```python
from build123d import *

# Parameters (mm, degrees)
SKETCH1_W            = 127
SKETCH1_H            = 25.4
BOSS_EXTRUDE1_DEPTH  = 4.7625
SKETCH2_W            = 4.7625
SKETCH2_H            = 25.4
SKETCH2_H_2          = 12.7
BOSS_EXTRUDE2_DEPTH  = 44.45
SKETCH3_W            = 25.4
SKETCH3_H            = 4.7625
BOSS_EXTRUDE3_DEPTH  = 7.9375
SKETCH4_W            = 12.7
SKETCH4_H            = 4.7625
BOSS_EXTRUDE4_DEPTH  = 7.9375
FILLET1_R            = 6.35
FILLET1_OF_MIRROR1_R = 6.35
SKETCH5_W            = 127
SKETCH5_H            = 2.0955
CUT_EXTRUDE1_DEPTH   = 5.08
SKETCH6_W            = 127
SKETCH6_H            = 1.5875
BOSS_EXTRUDE5_DEPTH  = 5.08


with BuildPart() as part:
    # Sketch1 → Boss-Extrude1 (new body)
    with BuildSketch(Plane(origin=(0, 0, 0), x_dir=(1, 0, 0), z_dir=(0, 1, 0))):
        with Locations((63.5, 12.7)):
            Rectangle(SKETCH1_W, SKETCH1_H)
    extrude(amount=BOSS_EXTRUDE1_DEPTH)

    # Sketch2 → Boss-Extrude2 (add)
    with BuildSketch(Plane(origin=(0, 4.7625, 0), x_dir=(1, 0, 0), z_dir=(0, 1, 0))):
        with Locations((42.06875, 12.7)):
            Rectangle(SKETCH2_W, SKETCH2_H)
        with Locations((16.66875, 6.35)):
            Rectangle(SKETCH2_W, SKETCH2_H_2)
    boss_extrude2 = extrude(amount=BOSS_EXTRUDE2_DEPTH)

    # Sketch3 → Boss-Extrude3 (add)
    with BuildSketch(Plane(origin=(44.45, 0, 0), x_dir=(0, 0, -1), z_dir=(1, 0, 0))):
        with Locations((12.7, 46.83125)):
            Rectangle(SKETCH3_W, SKETCH3_H)
    boss_extrude3 = extrude(amount=BOSS_EXTRUDE3_DEPTH)

    # Sketch4 → Boss-Extrude4 (add)
    with BuildSketch(Plane(origin=(19.05, 0, 0), x_dir=(0, 0, -1), z_dir=(1, 0, 0))):
        with Locations((6.35, 46.83125)):
            Rectangle(SKETCH4_W, SKETCH4_H)
    boss_extrude4 = extrude(amount=BOSS_EXTRUDE4_DEPTH)

    # Fillet1
    fillet1_edges = [part.edges().sort_by_distance(p)[0] for p in [
        (39.6875, 4.7625, -12.7),
        (44.45, 4.7625, -12.7),
        (19.05, 4.7625, -6.35),
        (14.2875, 4.7625, -6.35),
        (44.45, 44.45, -12.7),
        (19.05, 44.45, -6.35),
    ]]
    fillet(fillet1_edges, radius=FILLET1_R)

    # Mirror1: Boss-Extrude2, Boss-Extrude3, Boss-Extrude4 across plane
    add(boss_extrude2.mirror(Plane(origin=(63.5, 0, 0), x_dir=(0, 0, 1), z_dir=(1, 0, 0))))
    add(boss_extrude3.mirror(Plane(origin=(63.5, 0, 0), x_dir=(0, 0, 1), z_dir=(1, 0, 0))))
    add(boss_extrude4.mirror(Plane(origin=(63.5, 0, 0), x_dir=(0, 0, 1), z_dir=(1, 0, 0))))

    # Fillet1 of Mirror1
    fillet1_of_mirror1_edges = [part.edges().sort_by_distance(p)[0] for p in [
        (87.3125, 4.7625, -12.7),
        (82.55, 4.7625, -12.7),
        (107.95, 4.7625, -6.35),
        (112.7125, 4.7625, -6.35),
        (82.55, 44.45, -12.7),
        (107.95, 44.45, -6.35),
    ]]
    fillet(fillet1_of_mirror1_edges, radius=FILLET1_OF_MIRROR1_R)

    # Sketch5 → Cut-Extrude1 (cut)
    with BuildSketch(Plane.XY):
        with Locations((63.5, 2.38125)):
            Rectangle(SKETCH5_W, SKETCH5_H)
    extrude(amount=-CUT_EXTRUDE1_DEPTH, mode=Mode.SUBTRACT)

    # Sketch6 → Boss-Extrude5 (add)
    with BuildSketch(Plane(origin=(0, 0, -25.4), x_dir=(-1, 0, 0), z_dir=(0, 0, -1))):
        with Locations((-63.5, 2.38125)):
            Rectangle(SKETCH6_W, SKETCH6_H)
    extrude(amount=BOSS_EXTRUDE5_DEPTH)


solid = part.part
```
CAD build for the part. Positions are in the model's coordinates, mm. A direction names the side the tool comes from. Round coordinates to 2 decimals unless told otherwise and drop trailing zeros. Write each loop counter-clockwise with the first axis right and the second up, starting at its lowest first coordinate (ties: lowest second). Pieces come first, ordered by that corner, then holes. Notation, with made-up numbers: (-8.5, 60) - (32.5, 60) arc R25 cw to (32.5, 81) - close; hole circle Ø3 at (9, 9.5). An arc over 180 degrees is marked (long way). Return JSON: item names as keys, results as strings. Group by question number.
Item 1: Probe probe 1 along X at (y, z) = (26, -12); probe 2 along Y at (x, z) = (29.5, -2); probe 3 along X at (y, z) = (22, -14). List the from-to ranges inside material, lowest first.
Item 2: Band-saw the part on C-C on x = 90. List the corners of the cut face in (y, z) (1 decimal), plus the area to 3 significant figures.
Item 3: Band-saw the part on B-B on z = -17. List the corners of the cut face in (x, y).
Item 4: Band-saw the part on A-A on x = 54.5. List the corners of the cut face in (y, z) (1 decimal).
Item 5: 3-axis set-ups, long thin cutter, end or side, ignore diameter. For faces 1 (the face through (107.95, 24, -6)), 2 (the face through (64, 4, -25.4)), 3 (the face through (112.712, 30, -6)): which of +Z, -Z, +X, -X, +Y, -Y reach the whole face in a straight line?
Item 6: Flat gauge pins, fed straight in: pin 1 Ø4 at (x, z) = (37, -24) entering from +Y; pin 2 Ø3 at (x, y) = (108, 44) entering from -Z; pin 3 Ø4 at (y, z) = (46.5, -6.5) entering from -X. Where does each tip first touch, or does it go through?
Resolved:
{
 "1": {"probe 1": "x = 14.29 to 19.05, 39.69 to 44.45, 82.55 to 87.31, 107.95 to 112.71", "probe 2": "y = 0 to 1.33, 3.43 to 4.76", "probe 3": "x = 39.69 to 44.45, 82.55 to 87.31"},
 "2": {"outline": "(0, -25.4) - (1.6, -25.4) - (1.6, -30.5) - (3.2, -30.5) - (3.2, -25.4) - (5.9, -25.4) - (5.9, 0) - (3.4, 0) - (3.4, -5.1) - (1.3, -5.1) - (1.3, 0) - (0, 0) - close", "area": "148 mm²"},
 "3": {"outline": "(0, 0) - (127, 0) - (127, 4.76) - (93.66, 4.76) arc R6.35 cw to (87.31, 11.11) - (87.31, 49.21) - (74.61, 49.21) - (74.61, 44.45) - (76.2, 44.45) arc R6.35 cw to (82.55, 38.1) - (82.55, 11.11) arc R6.35 cw to (76.2, 4.76) - (50.8, 4.76) arc R6.35 cw to (44.45, 11.11) - (44.45, 38.1) arc R6.35 cw to (50.8, 44.45) - (52.39, 44.45) - (52.39, 49.21) - (39.69, 49.21) - (39.69, 11.11) arc R6.35 cw to (33.34, 4.76) - (0, 4.76) - close"},
 "4": {"outline": "(0, -25.4) - (1.6, -25.4) - (1.6, -30.5) - (3.2, -30.5) - (3.2, -25.4) - (4.8, -25.4) - (4.8, 0) - (3.4, 0) - (3.4, -5.1) - (1.3, -5.1) - (1.3, 0) - (0, 0) - close"},
 "5": {"face 1": "+Z, -Z", "face 2": "-Z, +X, -X, +Y", "face 3": "+Z, -Z, +X, +Y"},
 "6": {"pin 1": "stops at y = 8.24", "pin 2": "stops at z = -12.7", "pin 3": "stops at x = 14.29"}
}
